Autodesk Inventor part; units mm, degrees
ref_plane "YZ Plane" through (0, 0, 0) normal (1, 0, 0) x (0, 1, 0)
ref_plane "XZ Plane" through (0, 0, 0) normal (0, 1, 0) x (-1, 0, 0)
ref_plane "XY Plane" through (0, 0, 0) normal (0, 0, 1) x (1, 0, 0)
sketch "Sketch1" plane through (0, 0, 0) normal (0, 0, 1) x (1, 0, 0)
  line L0 (-10, -10) -> (10, -10) construction
  line L1 (10, -10) -> (10, 10) construction
  line L2 (10, 10) -> (-10, 10) construction
  line L3 (-10, 10) -> (-10, -10) construction
  line L4 (-10, -10) -> (10, 10) construction
  line L5 (10, -10) -> (-10, 10) construction
  line L6 (10, -7.5) -> (-10, -7.5) construction
  line L7 (-10, -7.5) -> (-10, 7.5) construction
  line L8 (-10, 7.5) -> (10, 7.5) construction
  line L9 (10, 7.5) -> (10, -7.5) construction
  line L10 (10, -7.5) -> (-10, 7.5) construction
  line L11 (-10, -7.5) -> (10, 7.5) construction
  line L12 (12.5, -10) -> (-12.5, -10)
  line L13 (-12.5, -10) -> (-12.5, 10)
  line L14 (-12.5, 10) -> (12.5, 10)
  line L15 (12.5, 10) -> (12.5, -10)
  line L16 (12.5, -10) -> (-12.5, 10) construction
  line L17 (-12.5, -10) -> (12.5, 10) construction
  line L18 (15, -12.5) -> (-15, -12.5)
  line L19 (-15, -12.5) -> (-15, 12.5)
  line L20 (-15, 12.5) -> (15, 12.5)
  line L21 (15, 12.5) -> (15, -12.5)
  line L22 (15, -12.5) -> (-15, 12.5) construction
  line L23 (-15, -12.5) -> (15, 12.5) construction
  point P0 (0, 0)
  dimension "d0" = 20
  dimension "d1" = 20
  dimension "d2" = 20
  dimension "d3" = 15
  dimension "d4" = 25
  dimension "d5" = 20
  dimension "d6" = 30
  dimension "d7" = 25
extrude "Extrusion1" add sketch "Sketch1" along normal blind 7.5 contours L12 L13 L14 L15
extrude "Extrusion2" add sketch "Sketch1" along normal blind 40
hole "Hole1" at (-10, 7.5, 0) at (10, 7.5, 0) at (10, -7.5, 0) at (-10, -7.5, 0) direction (0, 0, 1) diameter 2.5 end through all both
fillet "Fillet1" radius 2.5 4 edges at (15, 12.5, 20) (-15, 12.5, 20) (15, -12.5, 20) (-15, -12.5, 20)
properties part number "slotcar_adapter"
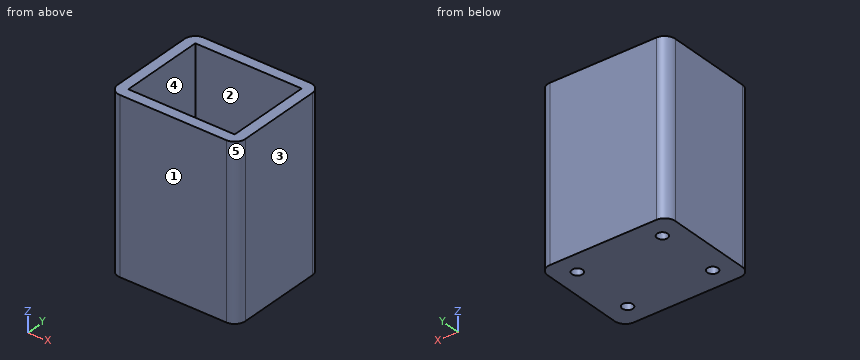
Verification items for the finished model (mm, model axes). Face numbers are marked on the shaded views. A direction names the side the tool comes from. Coordinates: 2 decimals unless noted, no trailing zeros. Loops run counter-clockwise (first coordinate to the right, second up) from the corner with the lowest first, then second, coordinate; pieces in that order, holes last. Notation, with made-up numbers: (33.5, 68.5) - (50.5, 68.5) arc R12 cw to (50.5, 82.5) - close; hole circle Ø1 at (62, 38). An arc over 180 degrees is marked (long way). Put each result on its own line as item: value.
Item 1: Section check D-D (z = 14.5). Enter the section's corners in (x, y), then the cut area to 3 significant figures.
Conclusion:
outline: (-15, -10) arc R2.5 ccw to (-12.5, -12.5) - (12.5, -12.5) arc R2.5 ccw to (15, -10) - (15, 10) arc R2.5 ccw to (12.5, 12.5) - (-12.5, 12.5) arc R2.5 ccw to (-15, 10) - close; hole (-12.5, -10) - (12.5, -10) - (12.5, 10) - (-12.5, 10) - close
area: 245 mm2
Item 2: Section check A-A (x = 10). Enter the section's corners in (y, z).
Conclusion:
outline: (-12.5, 0) - (-8.75, 0) - (-8.75, 7.5) - (-10, 7.5) - (-10, 40) - (-12.5, 40) - close; (-6.25, 0) - (6.25, 0) - (6.25, 7.5) - (-6.25, 7.5) - close; (8.75, 0) - (12.5, 0) - (12.5, 40) - (10, 40) - (10, 7.5) - (8.75, 7.5) - close
Item 3: Draft check along Y on the marked faces 1, 2 and 3. Enter one of: pulls with the +Y half, pulls with the -Y half, needs draft (parallel to the pull), parting line crosses it, or undercut.
Conclusion:
face 1: pulls with the -Y half
face 2: undercut
face 3: needs draft
Item 4: Section check C-C (y = -7.5). Enter the section's corners in (x, z).
Conclusion:
outline: (-15, 0) - (-11.25, 0) - (-11.25, 7.5) - (-12.5, 7.5) - (-12.5, 40) - (-15, 40) - close; (-8.75, 0) - (8.75, 0) - (8.75, 7.5) - (-8.75, 7.5) - close; (11.25, 0) - (15, 0) - (15, 40) - (12.5, 40) - (12.5, 7.5) - (11.25, 7.5) - close
Item 5: Set-up check for the marked faces 4 and 5: record each of +Z, -Z, +X, -X, +Y, -Y from which the full face is reachable in a straight line by a thin tool's end or side.
Conclusion:
face 4: +Z
face 5: +Z, -Z, +X, -Y
Item 6: Section check B-B (z = 7). Enter the section's corners in (x, y), then the cut area to 3 significant figures.
Conclusion:
outline: (-15, -10) arc R2.5 ccw to (-12.5, -12.5) - (12.5, -12.5) arc R2.5 ccw to (15, -10) - (15, 10) arc R2.5 ccw to (12.5, 12.5) - (-12.5, 12.5) arc R2.5 ccw to (-15, 10) - close; hole circle Ø2.5 at (-10, -7.5); hole circle Ø2.5 at (-10, 7.5); hole circle Ø2.5 at (10, -7.5); hole circle Ø2.5 at (10, 7.5)
area: 725 mm2
Item 7: Scan lines: line 1 along X through (y, z) = (-7.5, 3.5); line 2 along Y through (x, z) = (10, 3.5); line 3 along Y through (x, z) = (-3.25, 35.5). Record each from-to range of solid material in increasing order.
Conclusion:
line 1: x = -15 to -11.25, -8.75 to 8.75, 11.25 to 15
line 2: y = -12.5 to -8.75, -6.25 to 6.25, 8.75 to 12.5
line 3: y = -12.5 to -10, 10 to 12.5
Item 8: Gauge pin test, flat ends, axial feed: pin 1 Ø2 at (x, y) = (-7.5, -4.5) entering from +Z; pin 2 Ø2 at (x, y) = (-10, 7.5) entering from -Z (1 decimal). Record the tip position at first contact, or that the pin passes through.
Conclusion:
pin 1: stops at z = 7.5
pin 2: passes through
